from build123d import *

# Parameters (mm, degrees)
F0_W     = 58.42
F0_H     = 69.85
F1_DEPTH = 1.61925
F2_R     = 1.651
F3_DEPTH = 25.4
F4_R     = 8.001
F5_DEPTH = 21.11375
F6_R     = 1.27


with BuildPart() as f1:
    # F0 (on Top) → F1 (new body)
    with BuildSketch(Plane.XY):
        Rectangle(F0_W, F0_H)
    extrude(amount=F1_DEPTH)

    # F2 (on face) → F3 (cut)
    with BuildSketch(Plane.XY.offset(1.61925)):
        with Locations((-26.035, -31.75)):
            Circle(F2_R)
        with Locations((26.035, -31.75)):
            Circle(F2_R)
        with Locations((-26.035, 31.75)):
            Circle(F2_R)
        with Locations((26.035, 31.75)):
            Circle(F2_R)
    extrude(amount=-F3_DEPTH, mode=Mode.SUBTRACT)

    # F4 (on face) → F5 (join)
    with BuildSketch(Plane.XY.offset(1.61925)):
        with Locations((-15.8115, -2.2225)):
            Circle(F4_R)
        with Locations((15.7988, -2.2225)):
            Circle(F4_R)
    extrude(amount=F5_DEPTH)

    # F6
    f6_edges = [f1.edges().sort_by_distance(p)[0] for p in [
        (-23.8125, -2.2225, 22.733),
        (7.7978, -2.2225, 22.733),
    ]]
    fillet(f6_edges, radius=F6_R)


solid = f1.part
Could you check a few things on this model? Use its own coordinates, in mm. A direction names the side the tool comes from. Give positions to 0.01 mm unless a question says otherwise; leave off trailing zeros. Order: outer loops, then holes, each group sorted by start corner. A loop starts at its lowest first (then second) coordinate and runs counter-clockwise, first axis right, second up. Notation, with made-up numbers: (-6, 88.25) -> (5, 88.25) arc R34 cw to (5, 123.25) -> close; hole circle Ø4 at (18, 10.5). An arc over 180 degrees is marked (long way). Answer in a Markdown table with one row per item. Add a question column.
Item 1: We'd pull the mould along Y, two halves only. Please class faces 3 (the flat face through (-29.21, 0, 1)), 4 (the flat face through (0, 34.925, 1)), 5 (the cylindrical face through (-24.46, -31.25, 0.82)): pulls with the +Y half, pulls with the -Y half, needs draft (parallel to the pull), parting line crosses it, or undercut.
Item 2: I'm going to push flat-ended pins straight in: P1, Ø12, axis at x = 17, z = 8, coming from the -Y side; P2, Ø4, axis at x = -9.5, z = 13.5, coming from the -Y side; P3, Ø2, axis at x = -26.035, y = 31.75, coming from the +Z side; P4, Ø1.5, axis at x = 8, y = 5, coming from the +Z side. Where does each tip first touch, or does it pass through?
Item 3: Imagine slicing it at B-B (z = 10). List the corners of the cut face in (x, y) for me, and give its area (3 significant figures).
Item 4: Imagine slicing it at D-D (y = 14). List the corners of the cut face in (x, z) for me.
Item 5: Please list where these lines run through material, in increasing order: probe 1 along Z at (x, y) = (-10.5, -27); probe 2 along X at (y, z) = (-9, 13.25); probe 3 along Y at (x, z) = (-19.5, 20.25).
Item 6: For faces 1 (the cylindrical face through (7.806, -1.871, 11.402)), 2 (the cylindrical face through (24.82, 32.87, 0.82)), which set-ups out of +Z, -Z, +X, -X, +Y, -Y let a thin tool reach every point of the face, with its end or its side?
Item 7: Imagine slicing it at A-A (y = -31.75). List the corners of the cut face in (x, z) for me.
Item 8: Imagine slicing it at C-C (x = -4.5). List the corners of the cut face in (y, z) for me (3 decimals), and give its area (3 significant figures).
Result:
| question | item | result |
|---|---|---|
| 1 | face 3 | needs draft |
| 1 | face 4 | pulls with the +Y half |
| 1 | face 5 | undercut |
| 2 | P1 | y = -10.22 |
| 2 | P2 | y = -8.96 |
| 2 | P3 | through |
| 2 | P4 | z = 1.62 |
| 3 | outline | circle Ø16 at (-15.81, -2.22); circle Ø16 at (15.8, -2.22) |
| 3 | area | 402 mm2 |
| 4 | outline | (-29.21, 0) -> (29.21, 0) -> (29.21, 1.62) -> (-29.21, 1.62) -> close |
| 5 | probe 1 | 0 to 1.62 |
| 5 | probe 2 | -20.06 to -11.56, 11.55 to 20.05 |
| 5 | probe 3 | -9.32 to 4.88 |
| 6 | face 1 | +Z |
| 6 | face 2 | +Z, -Z |
| 7 | outline | (-29.21, 0) -> (-27.69, 0) -> (-27.69, 1.62) -> (-29.21, 1.62) -> close; (-24.38, 0) -> (24.38, 0) -> (24.38, 1.62) -> (-24.38, 1.62) -> close; (27.69, 0) -> (29.21, 0) -> (29.21, 1.62) -> (27.69, 1.62) -> close |
| 8 | outline | (-34.925, 0) -> (34.925, 0) -> (34.925, 1.619) -> (-34.925, 1.619) -> close |
| 8 | area | 113 mm2 |
